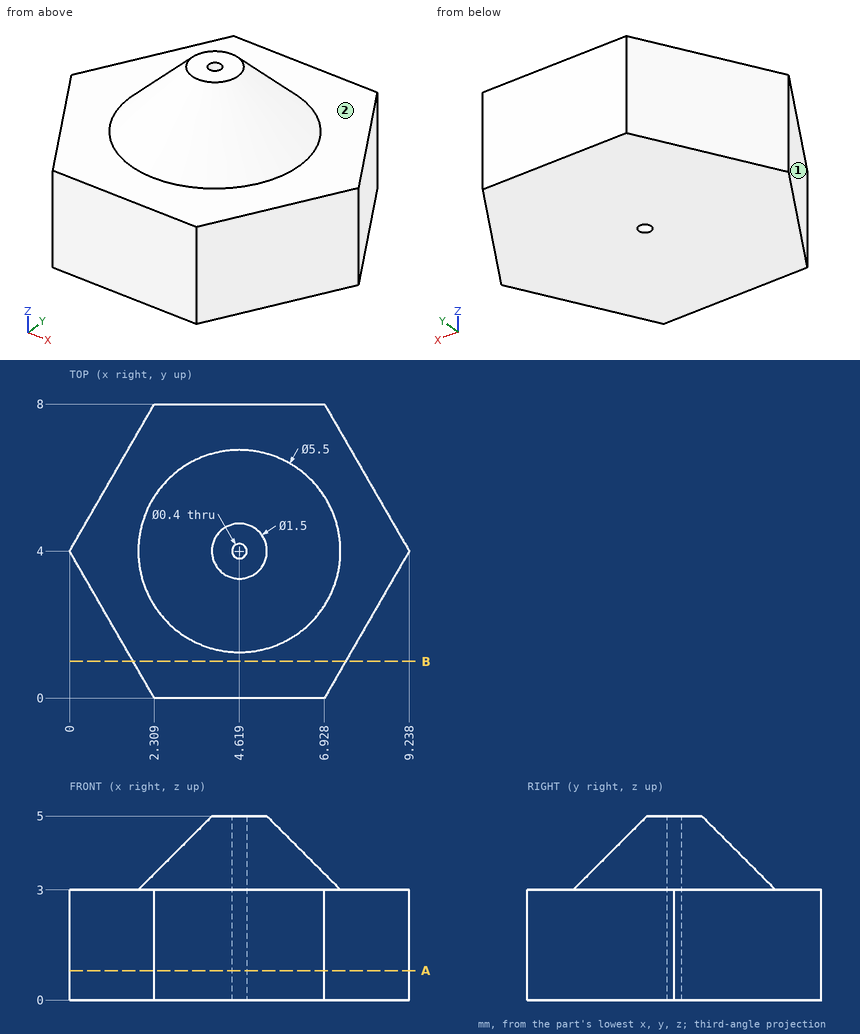
Could you check a few things on this drawing? It's one solid part, dimensions in mm from its lowest x, y, z. A direction names the side the tool comes from. Round coordinates to 2 decimals unless told otherwise and drop trailing zeros. Write each loop counter-clockwise with the first axis right and the second up, starting at its lowest first coordinate (ties: lowest second). Pieces come first, ordered by that corner, then holes. Notation, with made-up numbers: (52, 67.5) -> (82, 67.5) arc R31 ccw to (82, 98.5) -> close; hole circle Ø3 at (71, 18.25). An arc over 180 degrees is marked (long way). One line per question, with ' | ' between items. Start each with the question number.
1) I'm going to push flat-ended pins straight in: P1, Ø1, axis at x = 7.5, z = 4, coming from the +Y side; P2, Ø2, axis at y = 6, z = 0.5, coming from the -X side. Where does each tip first touch, or does it pass through?
2) I need wall thicknesses on line 1 (Z direction, x = 1.25, y = 3.25); line 2 (Y direction, x = 5, z = 4.25); line 3 (Z direction, x = 3, y = 2.75) (1 decimal). Which ranges of each line are inside material? Lowest first, please. Write a range as [from, to].
3) Suppose I cut it at A-A on z = 0.8. Write out the boundary of the cut face in (x, y), then the cut area to 3 significant figures.
4) Suppose I cut it at B-B on y = 1. Write out the boundary of the cut face in (x, z) (1 decimal), then the cut area to 3 significant figures.
5) On a 3-axis mill with a long thin cutter (end or side, diameter ignored), from which of +Z, -Z, +X, -X, +Y, -Y can I reach the whole of each face in a straight line? I mean the marked faces 1 and 2. Say none if no direction works.
Return value:
1) P1: passes through | P2: stops at x = 0.58
2) line 1: z = [0, 3] | line 2: y = [2.55, 5.45] | line 3: z = [0, 3.7]
3) outline: (0, 4) -> (2.31, 0) -> (6.93, 0) -> (9.24, 4) -> (6.93, 8) -> (2.31, 8) -> close; hole circle Ø0.4 at (4.62, 4) | area: 55.3 mm2
4) outline: (1.7, 0) -> (7.5, 0) -> (7.5, 3) -> (1.7, 3) -> close | area: 17.3 mm2
5) face 1: +Z, -Z, -X, -Y | face 2: +Z
